Part model, mm, in its own coordinate system. A direction names the side the tool comes from. Coordinates: 2 decimals unless noted, no trailing zeros. Loops run counter-clockwise (first coordinate to the right, second up) from the corner with the lowest first, then second, coordinate; pieces in that order, holes last. Notation, with made-up numbers: M -16,-36 L 15,-36 A18 ccw 15,-10 Z; hole C 42,34 d5. An arc over 180 degrees is marked long. Answer as a JSON object with one key per item and string values. Group by question number.
1. 3-axis set-ups, long thin cutter, end or side, ignore diameter. For faces 1 (the face through (0.54, 2.44, -18.65)), 2 (the face through (7.624, -0.094, -8.825)), 3 (the face through (5, 0, 4)): which of +Z, -Z, +X, -X, +Y, -Y reach the whole face in a straight line?
2. Saw through at B-B on x = 0. Write the cut outline in (y, z).
3. Drop flat-ended pins along their axis: pin 1 Ø3 at (x, z) = (3, -0.5) entering from +Y; pin 2 Ø4 at (x, y) = (3, -3) entering from +Z; pin 3 Ø0.5 at (x, y) = (5.5, 0) entering from +Z; pin 4 Ø2 at (x, y) = (1.5, 1.5) entering from +Z. Give the stop position or say it passes through.
4. Saw through at C-C on z = 13.5. Write the cut outline in (x, y), then the cut area to 3 significant figures.
5. Mould opens along Y. For faces 4 (the face through (-4.715, -0.326, 9.07)), 5 (the face through (-7.624, 0.094, -8.825)), 6 (the face through (3.4, -1.7, 14)) say: released by +Y, released by -Y, zero draft, split by the parting line, or undercut.
6. Saw through at D-D on z = 19. Write the cut outline in (x, y), then the cut area to 3 significant figures.
7. Drill centre lines: L1, parallel to Z at x = -2, y = 5; L2, parallel to Y at x = 5.5, z = 7.5; L3, parallel to Y at x = 2.5, z = -4.5. Where is each one in solid material? Low to high.
Autodesk Inventor part; units mm, degrees
ref_plane "YZ Plane" through (0, 0, 0) normal (1, 0, 0) x (0, 1, 0)
ref_plane "XZ Plane" through (0, 0, 0) normal (0, 1, 0) x (-1, 0, 0)
ref_plane "XY Plane" through (0, 0, 0) normal (0, 0, 1) x (1, 0, 0)
sketch "Sketch1" plane through (0, 0, 0) normal (0, 0, 1) x (1, 0, 0)
  circle A0 centre (0, 0) radius 8
  dimension "d0" = 16
extrude "Extrusion1" add sketch "Sketch1" along normal blind 14
sketch "Sketch2" plane through (0, 0, 14) normal (0, 0, 1) x (1, 0, 0)
  circle A0 centre (0, 0) radius 8
  circle A1 centre (5.5, 0) radius 0.85
  circle A2 centre (-5.5, 0) radius 0.85
  dimension "d3" = 1.7
  dimension "d4" = 1.7
  dimension "d5" = 5.5
  dimension "d6" = 5.5
extrude "Extrusion2" cut sketch "Sketch2" against normal blind 10 contours A1 | A2
sketch "Sketch3" plane through (0, 0, 14) normal (0, 0, 1) x (1, 0, 0)
  circle A0 centre (0, 0) radius 8
  circle A1 centre (0, 0) radius 3.5
  dimension "d9" = 7
extrude "Extrusion3" add sketch "Sketch3" along normal blind 2 contours A1
sketch "Sketch4" plane through (0, 0, 16) normal (0, 0, 1) x (1, 0, 0)
  circle A0 centre (0, 0) radius 3.5
  circle A1 centre (0, 0) radius 1.5
  dimension "d12" = 3
extrude "Extrusion4" add sketch "Sketch4" along normal blind 7.75 contours A1
sketch "Sketch5" plane through (0, 0, 0) normal (0, 0, -1) x (-1, 0, 0)
  circle A0 centre (0, 0) radius 8
  line L0 (-4.8302, 5.9) -> (4.8302, 5.9)
  line L1 (-4.8302, -5.9) -> (4.8302, -5.9)
  arc A1 (-4.8302, 5.9) -> (-4.8302, -5.9) centre (0, 0) ccw
  arc A2 (4.8302, -5.9) -> (4.8302, 5.9) centre (0, 0) ccw
  dimension "d16" = 5.9
  dimension "d17" = 5.9
extrude "Extrusion5" add sketch "Sketch5" along normal blind 18.4 contours L0 A2 L1 A1
fillet "Fillet1" radius 0.5 4 edges at (0, 5.9, -18.4) (7.625, 0, -18.4) (-7.625, 0, -18.4) (0, -5.9, -18.4)
sketch "Sketch6" plane through (0, 0, -18.4) normal (0, 0, -1) x (-1, 0, 0)
  arc A0 (-4.6482, 5.4) -> (-4.6482, -5.4) centre (0, 0) ccw
  circle A1 centre (0, 0) radius 2.5
  dimension "d21" = 5
extrude "Extrusion6" add sketch "Sketch6" along normal blind 0.5
properties part number "Gantry Motor"
Outcome:
{
 "1": {"face 1": "-Z", "face 2": "-Z, +X", "face 3": "+Z"},
 "2": {"outline": "M -8,0 L -5.9,0 L -5.9,-17.9 A0.5 ccw -5.4,-18.4 L -2.5,-18.4 L -2.5,-18.9 L 2.5,-18.9 L 2.5,-18.4 L 5.4,-18.4 A0.5 ccw 5.9,-17.9 L 5.9,0 L 8,0 L 8,14 L 3.5,14 L 3.5,16 L 1.5,16 L 1.5,23.75 L -1.5,23.75 L -1.5,16 L -3.5,16 L -3.5,14 L -8,14 Z"},
 "3": {"pin 1": "stops at y = 7.84", "pin 2": "stops at z = 16", "pin 3": "stops at z = 4", "pin 4": "stops at z = 23.75"},
 "4": {"outline": "C 0,0 d16; hole C -5.5,0 d1.7; hole C 5.5,0 d1.7", "area": "197 mm²"},
 "5": {"face 4": "undercut", "face 5": "split by the parting line", "face 6": "zero draft"},
 "6": {"outline": "C 0,0 d3", "area": "7.07 mm²"},
 "7": {"L1": "z = -18.4 to 14", "L2": "y = -5.81 to -0.85, 0.85 to 5.81", "L3": "y = -5.9 to 5.9"}
}
